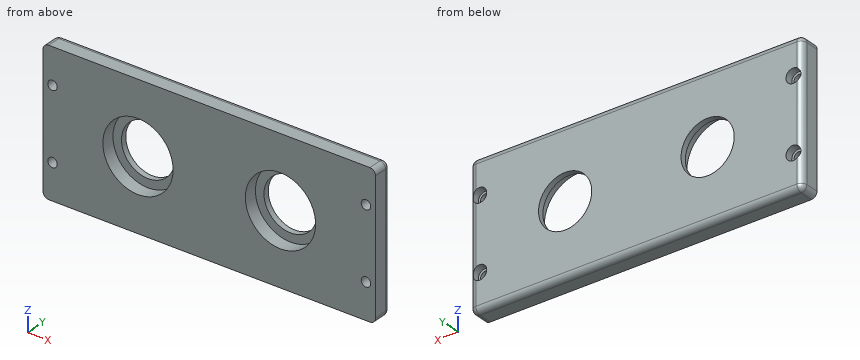
```python
from build123d import *

# Parameters (mm, degrees)
SKETCH1_W           = 175
SKETCH1_H           = 75
BOSS_EXTRUDE1_DEPTH = 10
SKETCH2_R           = 3.75
CUT_EXTRUDE1_DEPTH  = 4
SKETCH3_R           = 2.5
CUT_EXTRUDE2_DEPTH  = 96.720948595
SKETCH4_R           = 14
CUT_EXTRUDE3_DEPTH  = 96.720948595
SKETCH5_R           = 18.5
CUT_EXTRUDE4_DEPTH  = 7
FILLET1_R           = 3


with BuildPart() as part:
    # Sketch1 → Boss-Extrude1 (new body)
    with BuildSketch(Plane(origin=(0, 0, 0), x_dir=(1, 0, 0), z_dir=(0, 1, 0))):
        Rectangle(SKETCH1_W, SKETCH1_H)
    extrude(amount=BOSS_EXTRUDE1_DEPTH)

    # Sketch2 → Cut-Extrude1 (cut)
    with BuildSketch(Plane(origin=(0, 10, 0), x_dir=(1, 0, 0), z_dir=(0, 1, 0))):
        with Locations(Location((-82.5, 18.75, 0), (0, 0, 270))):
            Circle(SKETCH2_R)
        with Locations(Location((-82.5, -18.75, 0), (0, 0, 90))):
            Circle(SKETCH2_R)
        with Locations(Location((82.5, -18.75, 0), (0, 0, 270))):
            Circle(SKETCH2_R)
        with Locations(Location((82.5, 18.75, 0), (0, 0, 90))):
            Circle(SKETCH2_R)
    extrude(amount=-CUT_EXTRUDE1_DEPTH, mode=Mode.SUBTRACT)

    # Sketch3 → Cut-Extrude2 (cut, through all)
    with BuildSketch(Plane(origin=(0, 10, 0), x_dir=(1, 0, 0), z_dir=(0, 1, 0))):
        with Locations(Location((-82.5, 18.75, 0), (0, 0, 270))):
            Circle(SKETCH3_R)
        with Locations(Location((-82.5, -18.75, 0), (0, 0, 90))):
            Circle(SKETCH3_R)
        with Locations(Location((82.5, -18.75, 0), (0, 0, 270))):
            Circle(SKETCH3_R)
        with Locations(Location((82.5, 18.75, 0), (0, 0, 90))):
            Circle(SKETCH3_R)
    extrude(amount=-CUT_EXTRUDE2_DEPTH, mode=Mode.SUBTRACT)

    # Sketch4 → Cut-Extrude3 (cut, through all)
    with BuildSketch(Plane(origin=(0, 10, 0), x_dir=(1, 0, 0), z_dir=(0, 1, 0))):
        with Locations(Location((-37.5, 0, 0), (0, 0, 270))):
            Circle(SKETCH4_R)
    cut_extrude3 = extrude(amount=-CUT_EXTRUDE3_DEPTH, mode=Mode.SUBTRACT)

    # Sketch5 → Cut-Extrude4 (cut)
    with BuildSketch(Plane.XZ):
        with Locations(Location((-37.5, 0, 0), (0, 0, 270))):
            Circle(SKETCH5_R)
    cut_extrude4 = extrude(amount=-CUT_EXTRUDE4_DEPTH, mode=Mode.SUBTRACT)

    # Mirror1: Cut-Extrude3, Cut-Extrude4 across plane
    add(cut_extrude3.mirror(Plane(origin=(0, 0, 0), x_dir=(0, 0, 1), z_dir=(1, 0, 0))), mode=Mode.SUBTRACT)
    add(cut_extrude4.mirror(Plane(origin=(0, 0, 0), x_dir=(0, 0, 1), z_dir=(1, 0, 0))), mode=Mode.SUBTRACT)

    # Fillet1
    # the kernel refuses this fillet: 3 mm, written as the material it takes off along each edge
    with BuildSketch(Plane(origin=(-84.5, 7, 34.5), x_dir=(0, 1, 0), z_dir=(-1, 0, 0))) as fillet1_piece_1_section:
        Polygon((0, 0), (FILLET1_R, 0), (FILLET1_R, -FILLET1_R), (0, -FILLET1_R), align=None)
    fillet1_piece_1 = extrude(amount=FILLET1_R, mode=Mode.PRIVATE)
    fillet1_piece_1 = fillet1_piece_1 - Plane(origin=(-84.5, 7, 34.5), x_dir=(0, -0.7071067811865475, -0.7071067811865475), z_dir=(-1, 0, 0)) * Sphere(FILLET1_R, mode=Mode.PRIVATE)
    add(fillet1_piece_1, mode=Mode.SUBTRACT)
    with BuildSketch(Plane(origin=(-84.5, 7, -34.5), x_dir=(-1, 0, 0), z_dir=(0, 0, -1))) as fillet1_piece_2_section:
        Polygon((0, 0), (FILLET1_R, 0), (FILLET1_R, FILLET1_R), (0, FILLET1_R), align=None)
    fillet1_piece_2 = extrude(amount=FILLET1_R, mode=Mode.PRIVATE)
    fillet1_piece_2 = fillet1_piece_2 - Plane(origin=(-84.5, 7, -34.5), x_dir=(0.7071067811865475, -0.7071067811865475, 0), z_dir=(0, 0, -1)) * Sphere(FILLET1_R, mode=Mode.PRIVATE)
    add(fillet1_piece_2, mode=Mode.SUBTRACT)
    with BuildSketch(Plane(origin=(84.5, 7, 34.5), x_dir=(0, 1, 0), z_dir=(1, 0, 0))) as fillet1_piece_3_section:
        Polygon((0, 0), (FILLET1_R, 0), (FILLET1_R, FILLET1_R), (0, FILLET1_R), align=None)
    fillet1_piece_3 = extrude(amount=FILLET1_R, mode=Mode.PRIVATE)
    fillet1_piece_3 = fillet1_piece_3 - Plane(origin=(84.5, 7, 34.5), x_dir=(0, -0.7071067811865475, -0.7071067811865475), z_dir=(1, 0, 0)) * Sphere(FILLET1_R, mode=Mode.PRIVATE)
    add(fillet1_piece_3, mode=Mode.SUBTRACT)
    with BuildSketch(Plane(origin=(84.5, 7, -34.5), x_dir=(1, 0, 0), z_dir=(0, 0, -1))) as fillet1_piece_4_section:
        Polygon((0, 0), (FILLET1_R, 0), (FILLET1_R, -FILLET1_R), (0, -FILLET1_R), align=None)
    fillet1_piece_4 = extrude(amount=FILLET1_R, mode=Mode.PRIVATE)
    fillet1_piece_4 = fillet1_piece_4 - Plane(origin=(84.5, 7, -34.5), x_dir=(-0.7071067811865475, -0.7071067811865475, 0), z_dir=(0, 0, -1)) * Sphere(FILLET1_R, mode=Mode.PRIVATE)
    add(fillet1_piece_4, mode=Mode.SUBTRACT)
    with BuildSketch(Plane(origin=(-87.5, 10, 34.5), x_dir=(0, -1, 0), z_dir=(0, 0, -1)), Plane(origin=(87.5, 10, -34.5), x_dir=(0, -1, 0), z_dir=(0, 0, 1))) as fillet1_piece_5:
        with BuildLine():
            CenterArc((FILLET1_R, -FILLET1_R), FILLET1_R, 90, 90)
            Line((0, -FILLET1_R), (0, 0))
            Line((0, 0), (FILLET1_R, 0))
        make_face()
    extrude(amount=69, mode=Mode.SUBTRACT)
    with BuildSketch(Plane(origin=(84.5, 10, 37.5), x_dir=(0, 0, -1), z_dir=(-1, 0, 0))) as fillet1_piece_6:
        with BuildLine():
            CenterArc((FILLET1_R, FILLET1_R), FILLET1_R, 180, 90)
            Line((0, FILLET1_R), (0, 0))
            Line((0, 0), (FILLET1_R, 0))
        make_face()
    extrude(amount=169, mode=Mode.SUBTRACT)
    with BuildSketch(Plane(origin=(87.5, -7.5, 37.5), x_dir=(0, 0, -1), z_dir=(0, 1, 0)), Plane(origin=(87.5, -7.5, -37.5), x_dir=(-1, 0, 0), z_dir=(0, 1, 0))) as fillet1_piece_7:
        with BuildLine():
            CenterArc((FILLET1_R, FILLET1_R), FILLET1_R, 180, 90)
            Line((0, FILLET1_R), (0, 0))
            Line((0, 0), (FILLET1_R, 0))
        make_face()
    extrude(amount=14.5, mode=Mode.SUBTRACT)
    with BuildSketch(Plane(origin=(-87.5, -7.5, 37.5), x_dir=(0, 0, -1), z_dir=(0, 1, 0)), Plane(origin=(-87.5, -7.5, -37.5), x_dir=(1, 0, 0), z_dir=(0, 1, 0))) as fillet1_piece_8:
        with BuildLine():
            CenterArc((FILLET1_R, -FILLET1_R), FILLET1_R, 90, 90)
            Line((0, -FILLET1_R), (0, 0))
            Line((0, 0), (FILLET1_R, 0))
        make_face()
    extrude(amount=14.5, mode=Mode.SUBTRACT)
    with BuildSketch(Plane(origin=(-84.5, 10, -37.5), x_dir=(0, -1, 0), z_dir=(1, 0, 0))) as fillet1_piece_9:
        with BuildLine():
            CenterArc((FILLET1_R, -FILLET1_R), FILLET1_R, 90, 90)
            Line((0, -FILLET1_R), (0, 0))
            Line((0, 0), (FILLET1_R, 0))
        make_face()
    extrude(amount=169, mode=Mode.SUBTRACT)


solid = part.part
```
Could you check a few things on this model? Use its own coordinates, in mm. Round coordinates to 2 decimals unless told otherwise and drop trailing zeros. Write each loop counter-clockwise with the first axis right and the second up, starting at its lowest first coordinate (ties: lowest second). Pieces come first, ordered by that corner, then holes. Notation, with made-up numbers: M 6,-25 L 22,-25 A15 cw 22,-15 Z; hole C 87.5,18 d11. An arc over 180 degrees is marked long. Write each question's results on one line, items separated by ' | '. Start each with the question number.
1. Imagine slicing it at C-C on y = 3.25. List the corners of the cut face in (x, z) for me, and give its area (3 significant figures).
2. I'm going to push flat-ended pins straight in: pin 1 Ø7 at (x, z) = (-82.5, -18.75) entering from +Y; pin 2 Ø18.5 at (x, z) = (30.5, 0) entering from -Y. Where does each tip first touch, or does it pass through?
3. Imagine slicing it at A-A on z = 0. List the corners of the cut face in (x, y) for me.
4. Imagine slicing it at B-B on x = 37.5. List the corners of the cut face in (y, z) for me.
5. I need wall thicknesses on L1, parallel to X at y = 1.95, z = -18.75; L2, parallel to X at y = 5.5, z = -14; L3, parallel to Z at x = -82.5, y = 7.9. Which ranges of each line are inside material? Lowest first, please. Write a range as from..to.
6. Imagine slicing it at D-D on x = -82.5. List the corners of the cut face in (y, z) for me.
Result sheet:
1) outline: M -87.5,-34.5 A3 ccw -84.5,-37.5 L 84.5,-37.5 A3 ccw 87.5,-34.5 L 87.5,34.5 A3 ccw 84.5,37.5 L -84.5,37.5 A3 ccw -87.5,34.5 Z; hole C -82.5,-18.75 d5; hole C -82.5,18.75 d5; hole C -37.5,0 d37; hole C 37.5,0 d37; hole C 82.5,-18.75 d5; hole C 82.5,18.75 d5 | area: 10,900 mm^2
2) pin 1: stops at y = 6 | pin 2: stops at y = 7
3) outline: M -87.5,0 L -56,0 L -56,7 L -51.5,7 L -51.5,10 L -84.5,10 A3 ccw -87.5,7 Z; M -23.5,7 L -19,7 L -19,0 L 19,0 L 19,7 L 23.5,7 L 23.5,10 L -23.5,10 Z; M 51.5,7 L 56,7 L 56,0 L 87.5,0 L 87.5,7 A3 ccw 84.5,10 L 51.5,10 Z
4) outline: M 0,-37.5 L 7,-37.5 A3 ccw 10,-34.5 L 10,-14 L 7,-14 L 7,-18.5 L 0,-18.5 Z; M 0,18.5 L 7,18.5 L 7,14 L 10,14 L 10,34.5 A3 ccw 7,37.5 L 0,37.5 Z
5) L1: x = -87.5..-85, -80..80, 85..87.5 | L2: x = -87.5..-49.59, -25.41..25.41, 49.59..87.5 | L3: z = -37.36..-22.5, -15..15, 22.5..37.36
6) outline: M 0,-37.5 L 7,-37.5 A3 ccw 10,-34.5 L 10,-22.5 L 6,-22.5 L 6,-21.25 L 0,-21.25 Z; M 0,-16.25 L 6,-16.25 L 6,-15 L 10,-15 L 10,15 L 6,15 L 6,16.25 L 0,16.25 Z; M 0,21.25 L 6,21.25 L 6,22.5 L 10,22.5 L 10,34.5 A3 ccw 7,37.5 L 0,37.5 Z
